Part model, mm, in its own coordinate system. Face numbers are marked on the shaded views. A direction names the side the tool comes from. Round coordinates to 2 decimals unless told otherwise and drop trailing zeros. Write each loop counter-clockwise with the first axis right and the second up, starting at its lowest first coordinate (ties: lowest second). Pieces come first, ordered by that corner, then holes. Notation, with made-up numbers: M -21,-17 L 27,-17 A13 ccw 27,-13 Z; hole C -35,7 d3. An arc over 180 degrees is marked long. Use one line per item in the form item = value. Start each with the question number.
Item 1: Cut at C-C, the plane x = 140. Give the cut face in (y, z), then the cut area to 3 significant figures.
Item 2: Mould opens along Z. For the marked faces 1, 2 and 3 say: +Z half, -Z half, draft (parallel to the pull), parting line (faces both ways), or undercut.
Item 3: Cut at A-A, the plane x = 62. Give the cut face in (y, z).
Item 4: Cut at B-B, the plane y = -7. Give the cut face in (x, z).
Item 5: Flat gauge pins, fed straight in: pin 1 Ø1.5 at (x, z) = (121, -16.5) entering from -Y; pin 2 Ø5 at (x, y) = (138.5, -61) entering from +Z; pin 3 Ø3 at (x, z) = (125, 23) entering from +Y; pin 4 Ø5 at (x, y) = (92.5, -11) entering from +Z. Where does each tip first touch, or does it go through?
Item 6: Which spindle directions (+Z, -Z, +X, -X, +Y, -Y) get a long thin tool onto all of the face, cutting with end or side? Do the marked faces 4, 5 and 6. Say none if no direction does.
Item 7: Probe L1, parallel to X at y = -58, z = 0; L2, parallel to Z at x = 101.6, y = -61; L3, parallel to X at y = -66, z = 0. List the from-to ranges inside material, lowest first.
Autodesk Inventor part; units mm, degrees
ref_plane "Work Plane1" through (101.6, 117.6212, 0) normal (0, 0, -1) x (0, 1, 0)
ref_plane "Work Plane2" through (105.1179, 118.7756, 0) normal (0, 1, 0) x (1, 0, 0)
ref_plane "YZ Plane" through (0, 0, 0) normal (1, 0, 0) x (0, 1, 0)
sketch "Sketch1" plane through (0, 0, 0) normal (0, 0, 1) x (1, 0, 0)
  line L0 (152.6339, -58.2676) -> (152.6339, -92.0496)
  line L1 (151.7318, -58.2676) -> (152.6339, -58.2676)
  line L2 (151.7318, -48.9712) -> (151.7318, -58.2676)
  line L3 (136.4664, -48.9712) -> (136.4664, -74.3712)
  line L4 (136.4664, -74.3712) -> (120.4816, -90.3561)
  line L5 (120.4816, -90.3561) -> (101.6, -90.3561)
  line L6 (101.6, -95.4786) -> (101.6, -90.3561)
  line L7 (116.0071, -95.4786) -> (101.6, -95.4786)
  line L8 (116.0071, -92.0496) -> (116.0071, -95.4786)
  line L9 (152.6339, -92.0496) -> (116.0071, -92.0496)
  line L10 (151.7318, -48.9712) -> (136.4664, -48.9712)
revolve "Revolution1" add sketch "Sketch1" angle 360 about axis through (101.6, -95.4786, 0) along (0, 1, 0)
sketch "Sketch2" plane through (101.6, -90.3561, 0) normal (0, 1, 0) x (1, 0, 0)
  circle A0 centre (0, 0) radius 14.4071
extrude "Extrusion1" add sketch "Sketch2" along normal blind 7.62
sketch "Sketch3" plane through (101.6, -82.7361, 0) normal (0, 1, 0) x (1, 0, 0)
  circle A0 centre (0, 0) radius 14.4071
  circle A1 centre (0, 0) radius 12.7
  dimension "d3" = 25.4
extrude "Extrusion2" add sketch "Sketch3" along normal blind 31.75 contours A1
sketch "Sketch4" plane through (101.6, -50.9861, 0) normal (0, 1, 0) x (1, 0, 0)
  circle A0 centre (0, 0) radius 12.7
  circle A1 centre (0, 0) radius 9.525
  dimension "d6" = 19.05
extrude "Extrusion3" add sketch "Sketch4" along normal blind 6.604 contours A1
sketch "Sketch6" plane through (101.6, -44.3821, 0) normal (0, 1, 0) x (1, 0, 0)
  circle A0 centre (0, 0) radius 9.525
  circle A1 centre (0, 0) radius 6.858
  dimension "d12" = 13.716
extrude "Extrusion5" add sketch "Sketch6" along normal blind 4.8768 contours A1
sketch "Sketch7" plane through (101.6, -39.5053, 0) normal (0, 1, 0) x (1, 0, 0)
  circle A0 centre (0, 0) radius 6.858
  circle A1 centre (0, 0) radius 7.9629
  dimension "d15" = 15.9258
extrude "Extrusion6" add sketch "Sketch7" along normal blind 0.6985 contours A0 | A1
sketch "Sketch8" plane through (101.6, -38.8068, 0) normal (0, 1, 0) x (1, 0, 0)
  circle A0 centre (0, 0) radius 7.9629
  circle A1 centre (0, 0) radius 5.1562
  dimension "d18" = 10.3124
extrude "Extrusion7" add sketch "Sketch8" along normal blind 7.8232 draft 30 contours A1
sketch "Sketch9" plane through (101.6, -30.9836, 0) normal (0, 1, 0) x (1, 0, 0)
  circle A0 centre (0, 0) radius 9.6729
  circle A1 centre (0, 0) radius 4.9784
  dimension "d21" = 9.9568
extrude "Extrusion8" add sketch "Sketch9" along normal blind 146.2532 contours A1
sketch "Sketch10" plane through (101.6, 115.2696, 0) normal (0, 1, 0) x (1, 0, 0)
  circle A0 centre (0, 0) radius 4.9784
  circle A1 centre (0, 0) radius 3.2639
  dimension "d24" = 6.5278
extrude "Extrusion9" add sketch "Sketch10" along normal blind 0.1925 contours A1
sketch "Sketch11" plane through (101.6, 115.4622, 0) normal (0, 1, 0) x (1, 0, 0)
  circle A0 centre (0, 0) radius 3.2639
  circle A1 centre (0, 0) radius 4.3688
  dimension "d27" = 8.7376
extrude "Extrusion10" add sketch "Sketch11" along normal blind 1.8796 contours A0 | A1
chamfer "Chamfer1" distance 0.1981 distance2 0.1981 1 edges at (97.2312, 117.3418, 0) measured on face at (105.9122, 116.7152, 0.7008)
chamfer "Chamfer2" distance 0.1981 distance2 0.1981 1 edges at (97.2312, 115.4622, 0) measured on face at (105.5266, 115.4622, 0.6089)
sketch "Sketch12" plane through (101.6, 117.3418, 0) normal (0, 1, 0) x (1, 0, 0)
  circle A0 centre (0, 0) radius 4.1707
  circle A1 centre (0, 0) radius 3.2385
  dimension "d34" = 6.477
extrude "Extrusion11" add sketch "Sketch12" along normal blind 0.2794 draft 45 contours A1
sketch "Sketch13" plane through (101.6, 117.6212, 0) normal (0, 1, 0) x (1, 0, 0)
  circle A0 centre (0, 0) radius 3.5179
extrude "Extrusion12" add sketch "Sketch13" along normal blind 0.2261
sketch "Sketch14" plane through (101.6, 117.8472, 0) normal (0, 1, 0) x (1, 0, 0)
  circle A0 centre (0, 0) radius 3.5179
extrude "Extrusion13" add sketch "Sketch14" along normal blind 2.0828
ref_plane "Work Plane1" through (101.6, 117.6212, 0) normal (0, 0, -1) x (0, 1, 0)
sketch "Sketch15" plane through (101.6, 117.6212, 0) normal (0, 0, -1) x (0, 1, 0)
  line L0 (0, 3.5179) -> (2.3089, 3.5179)
  line L1 (1.1544, 3.5179) -> (1.1544, 4.8361)
  circle A0 centre (1.1544, 4.8361) radius 1.7414
ref_plane "Work Plane2" through (105.1179, 118.7756, 0) normal (0, 1, 0) x (1, 0, 0)
sketch "Sketch16" plane through (105.1179, 118.7756, 0) normal (0, 1, 0) x (1, 0, 0)
  circle A0 centre (-3.5179, 0) radius 3.5179
sweep "Sweep1" cut profiles "Sketch15" path "Sketch16"
sketch "Sketch17" plane through (101.6, 119.93, 0) normal (0, 1, 0) x (1, 0, 0)
  circle A0 centre (0, 0) radius 3.5179
extrude "Extrusion14" add sketch "Sketch17" along normal blind 1.143
chamfer "Chamfer3" distance 0.2286 distance2 0.2286 1 edges at (98.0821, 121.073, 0) measured on face at (105.0723, 120.3, 0.5643)
sketch "Sketch18" plane through (101.6, 121.073, 0) normal (0, 1, 0) x (1, 0, 0)
  circle A0 centre (0, 0) radius 3.2893
  circle A1 centre (0, 0) radius 1.8372
  dimension "d48" = 3.6744
extrude "Extrusion15" add sketch "Sketch18" along normal blind 1.4478 contours A1
chamfer "Chamfer4" distance 0.4318 distance2 0.2286 1 edges at (99.7628, 122.5208, 0) measured on face at (101.0889, 122.0382, -1.7647)
sketch "Sketch19" plane through (101.6, 122.5208, 0) normal (0, 1, 0) x (1, 0, 0)
  circle A0 centre (0, 0) radius 1.6086
  circle A1 centre (0, 0) radius 1.5875
  dimension "d53" = 3.175
extrude "Extrusion16" add sketch "Sketch19" along normal blind 11.3284 contours A1
sketch "Sketch20" plane through (101.6, 133.8492, 0) normal (0, 1, 0) x (1, 0, 0)
  circle A0 centre (0, 0) radius 1.5875
extrude "Extrusion17" add sketch "Sketch20" along normal blind 4.2164 draft -20
properties part number "plunger"
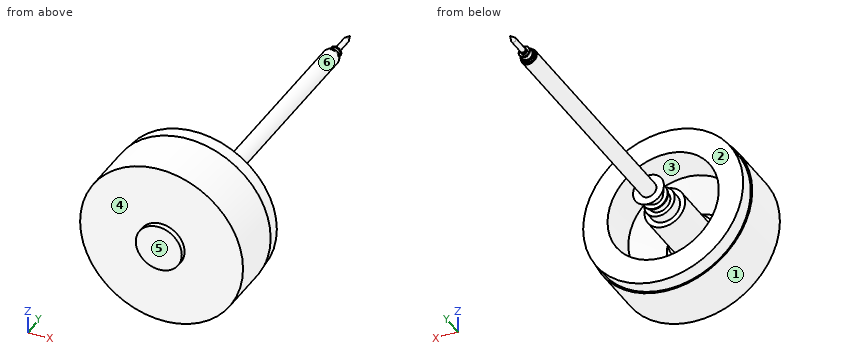
Model answer:
q1.outline = M -92.05,-33.61 L -58.27,-33.61 L -58.27,-32.23 L -48.97,-32.23 L -48.97,32.23 L -58.27,32.23 L -58.27,33.61 L -92.05,33.61 Z
q1.area = 2,870 mm²
q2.face_1 = parting line
q2.face_2 = draft
q2.face_3 = undercut
q3.outline = M -92.05,-32.19 L -58.27,-32.19 L -58.27,-30.74 L -48.97,-30.74 L -48.97,30.74 L -58.27,30.74 L -58.27,32.19 L -92.05,32.19 Z
q4.outline = C 101.6,0 d9.96
q5.pin_1 = -92.05
q5.pin_2 = 37.7
q5.pin_3 = -74.93
q5.pin_4 = through
q6.face_4 = -Y
q6.face_5 = +Z, -Z, +X, -X, -Y
q6.face_6 = +Y
q7.L1 = 51.47 to 66.73, 88.9 to 114.3, 136.47 to 151.73
q7.L2 = -51.03 to -34.87, -12.7 to 12.7, 34.87 to 51.03
q7.L3 = 50.57 to 66.73, 88.9 to 114.3, 136.47 to 152.63
